Study the drawing (mm; zero at the part's minimum x, y, z) and answer. Round coordinates to 2 decimals unless told otherwise and drop trailing zeros. Order: outer loops, then holes, each group sorted by start corner. A loop starts at its lowest first (then second) coordinate and runs counter-clockwise, first axis right, second up. Notation, with made-up numbers: (-12.5, -21.75) - (21.5, -21.75) arc R22 cw to (21.5, -6.75) - close; hole circle Ø2 at (-2, -35.5). An arc over 180 degrees is marked (long way). Put each result on its own line as item: value.
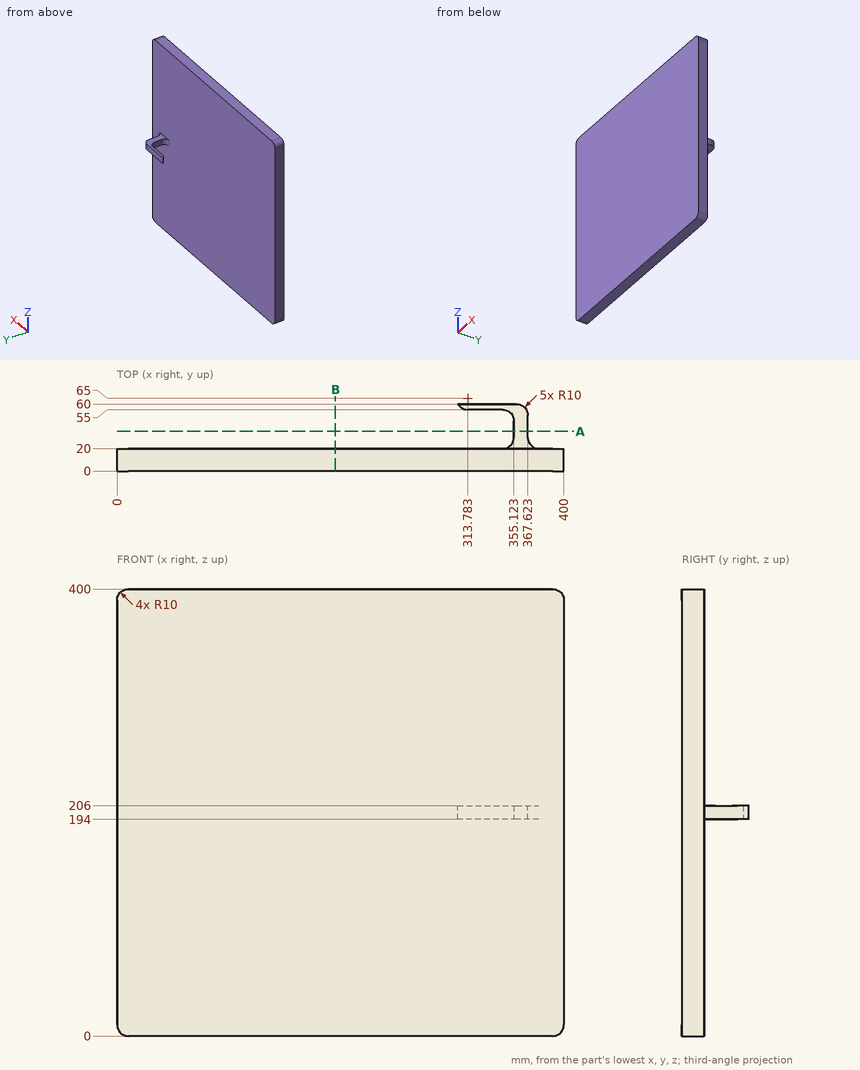
1) A cutting plane is placed at B-B on x = 195.5. Write down the section's boundary in (y, z).
Findings below:
outline: (0, 0) - (20, 0) - (20, 400) - (0, 400) - close
2) Given pin 1 Ø10 at (x, z) = (136, 45.5) entering from +Y; pin 2 Ø9.5 at (y, z) = (41.5, 197.5) entering from +X; pin 3 Ø10 at (x, y) = (358.5, 46.5) entering from +Z; pin 4 Ø20 at (x, y) = (336, 33) entering from +Z, each flat-ended and moving along its own axis, determine where each tip first touches the part or whether it passes through.
Findings below:
pin 1: stops at y = 20
pin 2: stops at x = 367.62
pin 3: stops at z = 206
pin 4: passes through
3) Straight lines are drawn through the part: L1, parallel to Y at x = 277, z = 25.5; L2, parallel to Z at x = 367, y = 23.5. For each, find the intervals that lie inside material, in ascending order. Write a range as from..to.
Findings below:
L1: y = 0..20
L2: z = 194..206
4) A cutting plane is placed at A-A on y = 35.5. Write down the section's boundary in (x, z), then the cut area to 3 significant figures.
Findings below:
outline: (355.12, 194) - (367.62, 194) - (367.62, 206) - (355.12, 206) - close
area: 150 mm2
